from build123d import *

# Parameters (mm, degrees)
SKETCH_1_R               = 1.5
SKETCH_1_R_2             = 2.1
EXTRUDE_1_DEPTH          = 105.25
FILLET_1_R               = 1
CUT_EXTRUDE_1_DEPTH      = 107.620835206
CUT_EXTRUDE_1_DEPTH_BACK = 107.620835206
SKETCH_2_R               = 2.05


with BuildPart() as part:
    # 草图1 → 凸台-拉伸1 (new, symmetric)
    with BuildSketch(Plane.XY):
        Polygon((-10, 10), (-10, 4.8), (-8.34, 3.14), (-8.34, 5.4), (-5.753553391, 5.4), (-3.8, 3.446446609), (-3.8, -3.446446609), (-5.753553391, -5.4), (-8.34, -5.4), (-8.34, -3.14), (-10, -4.8), (-10, -10), (-4.8, -10), (-3.14, -8.34), (-5.4, -8.34), (-5.4, -5.753553391), (-3.446446609, -3.8), (3.446446609, -3.8), (5.4, -5.753553391), (5.4, -8.34), (3.14, -8.34), (4.8, -10), (10, -10), (10, -4.8), (8.34, -3.14), (8.34, -5.4), (5.753553391, -5.4), (3.8, -3.446446609), (3.8, 3.446446609), (5.753553391, 5.4), (8.34, 5.4), (8.34, 3.14), (10, 4.8), (10, 10), (4.8, 10), (3.14, 8.34), (5.4, 8.34), (5.4, 5.753553391), (3.446446609, 3.8), (-3.446446609, 3.8), (-5.4, 5.753553391), (-5.4, 8.34), (-3.14, 8.34), (-4.8, 10), align=None)
        with Locations(Location((-7.5, 7.5, 0), (0, 0, 180))):
            Circle(SKETCH_1_R, mode=Mode.SUBTRACT)
        with Locations(Location((0, 0, 0), (0, 0, 180))):
            Circle(SKETCH_1_R_2, mode=Mode.SUBTRACT)
        with Locations(Location((-7.5, -7.5, 0), (0, 0, 180))):
            Circle(SKETCH_1_R, mode=Mode.SUBTRACT)
        with Locations(Location((7.5, -7.5, 0), (0, 0, 180))):
            Circle(SKETCH_1_R, mode=Mode.SUBTRACT)
        with Locations(Location((7.5, 7.5, 0), (0, 0, 180))):
            Circle(SKETCH_1_R, mode=Mode.SUBTRACT)
    extrude(amount=EXTRUDE_1_DEPTH, both=True)

    # 圆角1
    fillet_1_edges = [part.edges().sort_by_distance(p)[0] for p in [
        (10, 10, 0),
        (10, -10, 0),
        (-10, -10, 0),
        (-10, 10, 0),
    ]]
    fillet(fillet_1_edges, radius=FILLET_1_R)

    # 草图2 → 切除-拉伸1 (cut, two sides: drawn at the far end of the back side and taken through both)
    with BuildSketch(Plane(origin=(0, 3.8, 0), x_dir=(1, 0, 0), z_dir=(0, 1, 0)).offset(-CUT_EXTRUDE_1_DEPTH_BACK)):
        with Locations(Location((0, -15.25, 0), (0, 0, 270))):
            Circle(SKETCH_2_R)
        with Locations(Location((0, -0.25, 0), (0, 0, 270))):
            Circle(SKETCH_2_R)
    extrude(amount=CUT_EXTRUDE_1_DEPTH + CUT_EXTRUDE_1_DEPTH_BACK, mode=Mode.SUBTRACT)


solid = part.part
Verification items for the finished model (mm, model axes). Give positions to 0.01 mm unless a question says otherwise; leave off trailing zeros. Order: outer loops, then holes, each group sorted by start corner. A loop starts at its lowest first (then second) coordinate and runs counter-clockwise, first axis right, second up. Notation, with made-up numbers: M 54,79.25 L 66,79.25 A28 cw 66,117.25 Z; hole C -29.75,41.25 d3. An arc over 180 degrees is marked long. Use one line per item in the form item = value. Start each with the question number.
Q1. Scan lines: line 1 along Z through (x, y) = (0, -2.55); line 2 along Y through (x, z) = (7.5, 17.5). Record each from-to range of solid material in increasing order. Write a range as [from, to].
Q2. Go/stop test with flat-tipped pins: pin 1 Ø5.5 at (x, z) = (0, 15.25) entering from +Y; pin 2 Ø2 at (y, z) = (-1.5, 30.5) entering from -X; pin 3 Ø1.1 at (x, z) = (4, -51.5) entering from -Y. Record where each tip stops, or that it passes through.
Q3. Mould release check, pull along X, two halves, no side actions. Record for faces 1 (the flat face through (2.3, 3.8, 1.5)), 2 (the flat face through (-7, -10, 1)), 3 (the flat face through (-10, 7, 1)): +X half, -X half, draft (parallel to the pull), parting line (faces both ways), or undercut.
Q4. Section check B-B (z = 0.25). Count the separate pieces of the cut face and the enclosed holes in it, then the cut area to 3 significant figures.
Q5. Section check A-A (x = 0). Enter the section's corners in (y, z), then the cut area to 3 significant figures.
Evaluation:
q1.line_1 = [-105.25, -1.8], [2.3, 13.2], [17.3, 105.25]
q1.line_2 = [-10, -9], [-6, -5.4], [5.4, 6], [9, 10]
q2.pin_1 = 3.8
q2.pin_2 = -3.8
q2.pin_3 = -9.75
q3.face_1 = undercut
q3.face_2 = draft
q3.face_3 = -X half
q4.separate_pieces = 2
q4.enclosed_holes = 4
q4.area = 106 mm2
q5.outline = M -3.8,-105.25 L -2.1,-105.25 L -2.1,-1.8 L -3.8,-1.8 Z; M -3.8,2.3 L -2.1,2.3 L -2.1,13.2 L -3.8,13.2 Z; M -3.8,17.3 L -2.1,17.3 L -2.1,105.25 L -3.8,105.25 Z; M 2.1,-105.25 L 3.8,-105.25 L 3.8,-1.8 L 2.1,-1.8 Z; M 2.1,2.3 L 3.8,2.3 L 3.8,13.2 L 2.1,13.2 Z; M 2.1,17.3 L 3.8,17.3 L 3.8,105.25 L 2.1,105.25 Z
q5.area = 688 mm2
